Read the model definition and answer for the solid it produces. Units are mm, in the model's axes. A direction names the side the tool comes from. Round coordinates to 2 decimals unless told otherwise and drop trailing zeros. Write each loop counter-clockwise with the first axis right and the second up, starting at its lowest first coordinate (ties: lowest second). Pieces come first, ordered by that corner, then holes. Notation, with made-up numbers: (-39, 87) - (8, 87) arc R23 ccw to (8, 108) - close; hole circle Ø11 at (86.5, 4.25). An arc over 180 degrees is marked (long way). Use one line per item in the form item = value. Start each with the question number.
1) The part is cut by section B-B, the plane z = 45.5. Give the vertices of the cut face in (x, y).
2) The part is cut by section D-D, the plane y = -5. Count the separate pieces of the cut face and the enclosed holes in it, plus the area to 3 significant figures.
3) Consider line 1 along X through (y, z) = (-5, 60.75); line 2 along Y through (x, z) = (5, 61); line 3 along X through (y, z) = (5, 4.5). Determine where each line is inside the solid, lowest interval first. Write a range as from..to.
4) Each of these flat-tipped pins is pushed along its axis until it touches: pin 1 (3.5 mm diameter, centred on x = 5, y = 5, fed in from -Z); pin 2 (12 mm diameter, centred on y = 7.5, z = 17, fed in from -X); pin 3 (10 mm diameter, centred on y = 0, z = 14, fed in from +X); pin 4 (4.5 mm diameter, centred on x = -25, y = -3.5, fed in from -Z). Where does it stop, or does it pass through?
5) For faces 4 (the face through (-12.496, 5.347, 58.162)), 5 (the face through (22.1, 0, 16)), 6 (the face through (-4, 0, 11.515)), determine the directions among +Z, -Z, +X, -X, +Y, -Y from which every point of the face is accessible in a straight line to the end or side of a thin tool.
6) The part is cut by section C-C, the plane z = 10. Give the vertices of the cut face in (x, y).
7) For a pull along Z with two mould halves and no side action, classify faces 1 (the face through (25, 0, 32)), 2 (the face through (17.5, 0, 32)), 3 (the face through (0, -10, 53)) as released by +Z, released by -Z, zero draft, split by the parting line, or undercut.
8) The part is cut by section A-A, the plane y = 0. Give the vertices of the cut face in (x, z), plus the area to 3 significant figures.
Autodesk Inventor part; units mm, degrees
ref_plane "YZ Plane" through (0, 0, 0) normal (1, 0, 0) x (0, 1, 0)
ref_plane "XZ Plane" through (0, 0, 0) normal (0, 1, 0) x (-1, 0, 0)
ref_plane "XY Plane" through (0, 0, 0) normal (0, 0, 1) x (1, 0, 0)
sketch "スケッチ1" plane through (0, 0, 0) normal (0, 0, 1) x (1, 0, 0)
  line L0 (-22.1, -10) -> (22.1, -10)
  line L1 (22.1, -10) -> (22.1, 10)
  line L2 (22.1, 10) -> (-22.1, 10)
  line L3 (-22.1, 10) -> (-22.1, -10)
  line L4 (-22.1, -10) -> (22.1, 10) construction
  line L5 (22.1, -10) -> (-22.1, 10) construction
  point P0 (0, 0)
  dimension "d0" = 44.2
  dimension "d1" = 20
extrude "押し出し1" add sketch "スケッチ1" along normal blind 32
sketch "スケッチ2" plane through (0, 0, 32) normal (0, 0, 1) x (1, 0, 0)
  line L0 (-27.8, -10) -> (27.8, -10)
  line L1 (27.8, -10) -> (27.8, 10)
  line L2 (27.8, 10) -> (-27.8, 10)
  line L3 (-27.8, 10) -> (-27.8, -10)
  line L4 (-27.8, -10) -> (27.8, 10) construction
  line L5 (27.8, -10) -> (-27.8, 10) construction
  point P0 (0, 0)
  dimension "d4" = 20
  dimension "d5" = 55.6
extrude "押し出し2" add sketch "スケッチ2" along normal blind 32
sketch "スケッチ3" plane through (0, 0, 0) normal (0, 1, 0) x (-1, 0, 0)
  line L0 (22.1, 0) -> (22.1, 32)
  line L1 (-17.5, 7.4854) -> (17.5, 7.4854)
  line L2 (17.5, 7.4854) -> (17.5, 56.5146)
  line L3 (17.5, 56.5146) -> (-17.5, 56.5146)
  line L4 (-17.5, 56.5146) -> (-17.5, 7.4854)
  line L5 (-17.5, 7.4854) -> (17.5, 56.5146) construction
  line L6 (17.5, 7.4854) -> (-17.5, 56.5146) construction
  line L7 (-17.5, 11.5146) -> (17.5, 11.5146)
  line L8 (17.5, 11.5146) -> (17.5, 52.4854)
  line L9 (17.5, 52.4854) -> (-17.5, 52.4854)
  line L10 (-17.5, 52.4854) -> (-17.5, 11.5146)
  line L11 (-17.5, 11.5146) -> (17.5, 52.4854) construction
  line L12 (17.5, 11.5146) -> (-17.5, 52.4854) construction
  point P0 (0, 0)
  point P1 (0, 32)
  dimension "d8" = 22.1
  dimension "d9" = 32
  dimension "d10" = 35
  dimension "d11" = 45
extrude "押し出し3" cut sketch "スケッチ3" against normal mid plane 32 contours L4 L9 L2 L7
sketch "スケッチ4" plane through (0, 0, 0) normal (0, 0, -1) x (-1, 0, 0)
  point P0 (0, 0)
  point P1 (0, 0)
hole "穴1" at (0, 0, 0) direction (0, 0, 1) diameter 6 depth 15 tip angle 118
sketch "スケッチ5" plane through (0, 0, 0) normal (0, 0, -1) x (-1, 0, 0)
  point P0 (0, 0)
  point P1 (-5, 5)
  point P2 (-5, -5)
  point P3 (5.0409, -5)
  point P4 (5, 5)
  dimension "d21" = 5
  dimension "d22" = 5
  dimension "d23" = 5
  dimension "d24" = 5
  dimension "d25" = 5.0409
  dimension "d26" = 5
hole "穴2" at (5, 5, 0) at (5, -5, 0) at (-5.0409, -5, 0) at (-5, 5, 0) direction (0, 0, 1) diameter 3.2 depth 15 tip angle 118
sketch "スケッチ6" plane through (0, 0, 64) normal (0, 0, 1) x (1, 0, 0)
  point P0 (0, 0)
  point P1 (0, 0)
hole "穴3" at (0, 0, 64) direction (0, 0, -1) diameter 6 depth 15 tip angle 118
sketch "スケッチ7" plane through (0, 0, 64) normal (0, 0, 1) x (1, 0, 0)
  circle A0 centre (-5.0409, -5) radius 1.6
  circle A1 centre (-5, 5) radius 1.6
  circle A2 centre (5, 5) radius 1.6
  circle A3 centre (5, -5) radius 1.6
  point P0 (0, 0)
  point P1 (-14.0582, -5)
  point P2 (-14.0582, 5)
  point P3 (13.4789, 5)
  point P4 (13.4789, -5)
hole "穴4" at (-5.0409, -5, 64) at (-5, 5, 64) at (5, 5, 64) at (5, -5, 64) at (-14.0582, -5, 64) at (-14.0582, 5, 64) at (13.4789, 5, 64) at (13.4789, -5, 64) direction (0, 0, -1) diameter 3.2 depth 17.1 tip angle 118
properties part number "20220612_サーボ仮"
Geometry results:
q1.outline = (-27.8, -10) - (-17.5, -10) - (-17.5, 10) - (-27.8, 10) - close; (17.5, -10) - (27.8, -10) - (27.8, 10) - (17.5, 10) - close
q2.separate_pieces = 6
q2.enclosed_holes = 0
q2.area = 1,540 mm2
q3.line_1 = -27.8..-15.66, -12.46..-6.64, -3.44..3.4, 6.6..11.88, 15.08..27.8
q3.line_2 = -10..-6.6, -3.4..3.4, 6.6..10
q3.line_3 = -22.1..-6.6, -3.4..3.4, 6.6..22.1
q4.pin_1 = 0
q4.pin_2 = -22.1
q4.pin_3 = 22.1
q4.pin_4 = 32
q5.face_4 = +Z
q5.face_5 = -Z, +X, +Y, -Y
q5.face_6 = +Y, -Y
q6.outline = (-22.1, -10) - (22.1, -10) - (22.1, 10) - (-22.1, 10) - close; hole circle Ø3.2 at (-5.04, -5); hole circle Ø3.2 at (-5, 5); hole circle Ø6 at (0, 0); hole circle Ø3.2 at (5, -5); hole circle Ø3.2 at (5, 5)
q7.face_1 = released by -Z
q7.face_2 = undercut
q7.face_3 = zero draft
q8.outline = (-27.8, 32) - (-22.1, 32) - (-22.1, 0) - (-3, 0) - (-3, 11.51) - (-17.5, 11.51) - (-17.5, 52.49) - (-3, 52.49) - (-3, 64) - (-27.8, 64) - close; (3, 0) - (22.1, 0) - (22.1, 32) - (27.8, 32) - (27.8, 64) - (3, 64) - (3, 52.49) - (17.5, 52.49) - (17.5, 11.51) - (3, 11.51) - close
q8.area = 1,620 mm2
